For this review, take the finished solid that the model builds, in its own axes (mm). A direction names the side the tool comes from. Round coordinates to 2 decimals unless told otherwise and drop trailing zeros. Order: outer loops, then holes, each group sorted by start corner. A loop starts at its lowest first (then second) coordinate and runs counter-clockwise, first axis right, second up. Notation, with made-up numbers: (11, -1) - (26, -1) arc R9 cw to (26, 7) - close; hole circle Ø8 at (38.25, 62.5). An arc over 180 degrees is marked (long way). One line per question, with ' | ' between items.
```python
from build123d import *

# Parameters (mm, degrees)
F0_W      = 74.5829641819
F0_H      = 30.8565702289
F1_DEPTH  = 25.4
F2_DEPTH  = 25.4
F3_DEPTH  = 25.4
F4_DEPTH  = 25.4
F6_DEPTH  = 25.4
F7_DEPTH  = 151.384
F8_DEPTH  = 25.4
F9_W      = 39.2481669128
F9_H      = 17.8465423578
F12_DEPTH = 60.198
F10_W     = 38.687005946
F10_H     = 16.2959610515
F13_DEPTH = 64.262
F14_DEPTH = 39.116
F15_DEPTH = 38.862
F16_DEPTH = 25.4
F17_DEPTH = 25.4
F19_DEPTH = 107.442
F21_DEPTH = 58.166
F22_DEPTH = 25.4
F23_DEPTH = 25.4
F24_DEPTH = 16.51
F25_DEPTH = 18.288
F26_R     = 11.2114596222
F27_DEPTH = 45.72
F28_R     = 10.9420459353
F29_DEPTH = 60.452


with BuildPart() as f1:
    # F0 (on Front) → F1 (new body)
    with BuildSketch(Plane.XZ):
        with Locations((-37.291482091, 15.4282851145)):
            Rectangle(F0_W, F0_H)
    extrude(amount=F1_DEPTH)

    # F2 (add): a face of the model
    f2_faces = [f1.faces().sort_by_distance(p)[0] for p in [
        (-74.5829641819, -12.7, 15.4282851145),
    ]]
    extrude(f2_faces, amount=F2_DEPTH)

    # F3 (add): a face of the model
    f3_faces = [f1.faces().sort_by_distance(p)[0] for p in [
        (-49.991482091, -12.7, 30.8565702289),
    ]]
    extrude(f3_faces, amount=F3_DEPTH)

    # F4 (add): a face of the model
    f4_faces = [f1.faces().sort_by_distance(p)[0] for p in [
        (-49.991482091, -25.4, 28.1282851145),
    ]]
    extrude(f4_faces, amount=F4_DEPTH)

    # F5 (on face) → F6 (cut)
    with BuildSketch(Plane(origin=(-99.9829641819, 0, 0), x_dir=(0, -1, 0), z_dir=(-1, 0, 0))):
        with BuildLine():
            ThreePointArc((0, 32.8871821457), (25.4, 56.0189424458), (50.8, 32.8871821457))
            Line((50.8, 32.8871821457), (50.8, 56.2565702289))
            Line((50.8, 56.2565702289), (0, 56.2565702289))
            Line((0, 56.2565702289), (0, 32.8871821457))
        make_face()
    extrude(amount=-F6_DEPTH, mode=Mode.SUBTRACT)

    # F7 (cut): a face of the model
    f7_faces = [f1.faces().sort_by_distance(p)[0] for p in [
        (-74.5829641819, -25.4, 56.0748599591),
    ]]
    extrude(f7_faces, amount=-F7_DEPTH, mode=Mode.SUBTRACT)

    # F8 (add): a face of the model
    f8_faces = [f1.faces().sort_by_distance(p)[0] for p in [
        (0, -25.4, 25.6193021496),
    ]]
    extrude(f8_faces, amount=F8_DEPTH)

    # F9 (on face) → F12 (cut)
    with BuildSketch(Plane.XZ.offset(50.8)):
        with Locations((-80.3588807255, 23.9639109668)):
            Rectangle(F9_W, F9_H)
    extrude(amount=-F12_DEPTH, mode=Mode.SUBTRACT)

    # F10 (on face) → F13 (cut)
    with BuildSketch(Plane.XZ.offset(50.8)):
        with Locations((6.056497027, 24.7392016199)):
            Rectangle(F10_W, F10_H)
    extrude(amount=-F13_DEPTH, mode=Mode.SUBTRACT)

    # F14 (cut): a face of the model
    f14_faces = [f1.faces().sort_by_distance(p)[0] for p in [
        (-99.9829641819, -25.4, 42.6317575384),
    ]]
    extrude(f14_faces, amount=-F14_DEPTH, mode=Mode.SUBTRACT)

    # F15 (cut): a face of the model
    f15_faces = [f1.faces().sort_by_distance(p)[0] for p in [
        (25.4, -25.4, 42.6317575384),
    ]]
    extrude(f15_faces, amount=-F15_DEPTH, mode=Mode.SUBTRACT)

    # F16 (add): a face of the model
    f16_faces = [f1.faces().sort_by_distance(p)[0] for p in [
        (-99.9829641819, -25.4, 7.520319894),
    ]]
    extrude(f16_faces, amount=F16_DEPTH)

    # F17 (add): a face of the model
    f17_faces = [f1.faces().sort_by_distance(p)[0] for p in [
        (25.4, -25.4, 8.2956105471),
    ]]
    extrude(f17_faces, amount=F17_DEPTH)

    # F18 (on face) → F19 (cut)
    with BuildSketch(Plane.YZ.offset(-13.287005946)):
        with BuildLine():
            Line((-35.7976081282, 32.8871821457), (-15.1284308589, 32.8871821457))
            ThreePointArc((-15.1284308589, 32.8871821457), (-25.4630194936, 41.1995819956), (-35.7976081282, 32.8871821457))
        make_face()
    extrude(amount=-F19_DEPTH, mode=Mode.SUBTRACT)

    # F20 (on face) → F21 (cut)
    with BuildSketch(Plane(origin=(-60.7347972691, 0, 0), x_dir=(0, -1, 0), z_dir=(-1, 0, 0))):
        with BuildLine():
            ThreePointArc((13.880819181, 32.8871821457), (25.4630194936, 21.3049818331), (37.0452198061, 32.8871821457))
            Line((37.0452198061, 32.8871821457), (35.7976081282, 32.8871821457))
            Line((35.7976081282, 32.8871821457), (15.1284308589, 32.8871821457))
            Line((15.1284308589, 32.8871821457), (13.880819181, 32.8871821457))
        make_face()
        with BuildLine():
            Line((35.7976081282, 32.8871821457), (37.0452198061, 32.8871821457))
            ThreePointArc((37.0452198061, 32.8871821457), (25.4630194936, 44.4693824582), (13.880819181, 32.8871821457))
            Line((13.880819181, 32.8871821457), (15.1284308589, 32.8871821457))
            Line((15.1284308589, 32.8871821457), (35.7976081282, 32.8871821457))
        make_face()
    extrude(amount=-F21_DEPTH, mode=Mode.SUBTRACT)

    # F22 (cut): a face of the model
    f22_faces = [f1.faces().sort_by_distance(p)[0] for p in [
        (-60.7347972691, -36.4214139672, 33.146168018),
    ]]
    extrude(f22_faces, amount=F22_DEPTH, mode=Mode.SUBTRACT)

    # F23 (cut): a face of the model
    f23_faces = [f1.faces().sort_by_distance(p)[0] for p in [
        (-60.7347972691, -36.4214139672, 33.146168018),
    ]]
    extrude(f23_faces, amount=-F23_DEPTH, mode=Mode.SUBTRACT)

    # F24 (cut): a face of the model
    f24_faces = [f1.faces().sort_by_distance(p)[0] for p in [
        (50.8, -25.4, 8.2956105471),
    ]]
    extrude(f24_faces, amount=-F24_DEPTH, mode=Mode.SUBTRACT)

    # F25 (cut): a face of the model
    f25_faces = [f1.faces().sort_by_distance(p)[0] for p in [
        (-125.3829641819, -25.4, 7.520319894),
    ]]
    extrude(f25_faces, amount=-F25_DEPTH, mode=Mode.SUBTRACT)

    # F26 (on face) → F27 (cut)
    with BuildSketch(Plane.XY.offset(16.5912210941)):
        with Locations((9.9650174379, -25.5547314882)):
            Circle(F26_R)
    extrude(amount=-F27_DEPTH, mode=Mode.SUBTRACT)

    # F28 (on face) → F29 (cut)
    with BuildSketch(Plane.XY.offset(15.0406397879)):
        with Locations((-85.4209959507, -26.1354632676)):
            Circle(F28_R)
    extrude(amount=-F29_DEPTH, mode=Mode.SUBTRACT)


solid = f1.part
```
(1) For probe 1 along X at (y, z) = (-25.5, 9.5); probe 2 along Z at (x, y) = (12.5, -6.5); probe 3 along X at (y, z) = (-20.5, 17.5), list the stretches that pass through material, from the lowest coordinate up. Write a range as [from, to].
Output values:
probe 1: [-107.09, -96.34], [-74.5, -1.25], [21.18, 34.29] | probe 2: [0, 16.59] | probe 3: [-60.73, -13.29]
(2) We need section A-A on y = -28.5. State the section outline as (x, z) points.
Output values:
outline: (-107.09, 0) - (-96.1, 0) - (-96.1, 15.04) - (-107.09, 15.04) - close; (-74.74, 0) - (-0.85, 0) - (-0.85, 16.59) - (-13.29, 16.59) - (-13.29, 21.71) - (-60.73, 21.71) - (-60.73, 15.04) - (-74.74, 15.04) - close; (-60.87, 44.06) - (-13.46, 44.06) - (-13.46, 55.83) - (-60.87, 55.83) - close; (20.78, 0) - (34.29, 0) - (34.29, 16.59) - (20.78, 16.59) - close
(3) Insertion check: pin 1 (11.5 mm diameter, centred on y = -13.5, z = 47, fed in from -X); pin 2 (5 mm diameter, centred on y = -43.5, z = 26.5, fed in from -X); pin 3 (10 mm diameter, centred on x = -85, y = -10.5, fed in from +Z); pin 4 (14 mm diameter, centred on y = -25.46, z = 32.89, fed in from +X). Each pin has a flat end and moves straight along its axis. Give the tip position at first contact, or say it passes through.
Output values:
pin 1: x = -60.87 | pin 2: x = -60.73 | pin 3: z = 15.04 | pin 4: through
(4) Mouldability with a two-part tool opening along Y and no side actions: class faces 5 (the cylindrical face through (-37.496, -25.928, 56.013)), 6 (the cylindrical face through (-37.41, -31.69, 42.653)), 7 (the flat face through (-13.462, -25, 45)) as released by +Y, released by -Y, zero draft, split by the parting line, or undercut.
Output values:
face 5: split by the parting line | face 6: undercut | face 7: zero draft
(5) We need section D-D on y = -46.5. State the section outline as (x, z) points.
Output values:
outline: (-107.09, 0) - (34.29, 0) - (34.29, 16.59) - (-13.29, 16.59) - (-13.29, 32.89) - (-13.46, 32.89) - (-13.46, 44.85) - (-60.87, 44.85) - (-60.87, 32.89) - (-60.73, 32.89) - (-60.73, 15.04) - (-107.09, 15.04) - close
(6) For faces 1 (the flat face through (-13.287, -26, 21)), 2 (the flat face through (-60.735, -26, 20)), 3 (the flat face through (-60.867, -25, 47)), 4 (the flat face through (-37, -50.8, 13)), list the 3-axis set-ups (+Z, -Z, +X, -X, +Y, -Y) from which the entire face can be reached by the end or side of a thin tool; tool diameter is ignored.
Output values:
face 1: +Z, +X, +Y, -Y | face 2: -X, +Y, -Y | face 3: +Z, -X, +Y, -Y | face 4: +Z, -Z, +X, -X, -Y
(7) We need section B-B on x = -23. State the section outline as (y, z) points.
Output values:
outline: (-50.8, 0) - (0, 0) - (0, 32.89) arc R25.51 ccw to (-50.8, 32.89) - close; hole circle Ø23.16 at (-25.46, 32.89)
(8) We need section C-C on z = 37.5. State the section outline as (x, y) points.
Output values:
outline: (-60.87, -49.93) - (-13.46, -49.93) - (-13.46, -36.09) - (-60.87, -36.09) - close; (-60.87, -14.84) - (-13.46, -14.84) - (-13.46, -0.87) - (-60.87, -0.87) - close
